Part model, mm, in its own coordinate system. Face numbers are marked on the shaded views. A direction names the side the tool comes from. Round coordinates to 2 decimals unless told otherwise and drop trailing zeros. Write each loop counter-clockwise with the first axis right and the second up, starting at its lowest first coordinate (ties: lowest second). Pieces come first, ordered by that corner, then holes.
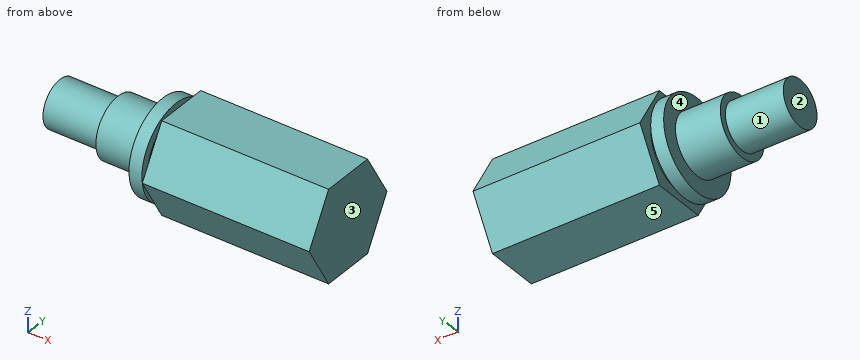
```python
from build123d import *

# Parameters (mm, degrees)
BOSS_EXTRUDE1_DEPTH = 22.86


with BuildPart() as part:
    # Sketch1 → Revolve1 (revolve)
    with BuildSketch(Plane.XY, mode=Mode.PRIVATE) as revolve1_sk:
        Polygon((0, 0), (0, 6.35), (-22.86, 6.35), (-22.86, 5.241687437), (-23.622, 5.241687437), (-23.622, 6.35), (-25.4, 6.35), (-25.4, 4.1275), (-31.5468, 4.1275), (-31.5468, 3.175), (-39.4843, 3.175), (-39.4843, 0), align=None)
    revolve(revolve1_sk.sketch.rotate(Axis((0, 0, 0), (-1, 0, 0)), 90), axis=Axis((0, 0, 0), (-1, 0, 0)))

    # Sketch2 → Boss-Extrude1 (add)
    with BuildSketch(Plane(origin=(0, 0, 0), x_dir=(0, 0, -1), z_dir=(1, 0, 0))):
        Polygon((-6.35, 3.666174209), (-6.35, -3.666174209), (0, -7.332348419), (6.35, -3.666174209), (6.35, 3.666174209), (0, 7.332348419), align=None)
    extrude(amount=-BOSS_EXTRUDE1_DEPTH)


solid = part.part
```
Q1. Wall check: L1, parallel to X at y = -5.5, z = 1; L2, parallel to X at y = 3.75, z = 0.25; L3, parallel to X at y = 1.75, z = 4.25. Give the ranges that are in metal, low to high.
Values follow:
L1: x = -25.4 to -23.62, -22.86 to 0
L2: x = -31.55 to 0
L3: x = -25.4 to 0
Q2. Which spindle directions (+Z, -Z, +X, -X, +Y, -Y) get a long thin tool onto all of the face, cutting with end or side? Do the marked faces 4 and 5. Say none if no direction does.
Values follow:
face 4: -X
face 5: -Z, +X, -X, +Y, -Y
Q3. Cut at C-C on z = -3.75. Write the cut outline in (x, y).
Values follow:
outline: (-31.55, -1.72) - (-25.4, -1.72) - (-25.4, -5.12) - (-23.62, -5.12) - (-23.62, -3.66) - (-22.86, -3.66) - (-22.86, -5.17) - (0, -5.17) - (0, 5.17) - (-22.86, 5.17) - (-22.86, 3.66) - (-23.62, 3.66) - (-23.62, 5.12) - (-25.4, 5.12) - (-25.4, 1.72) - (-31.55, 1.72) - close
Q4. Mould opens along X. For the marked faces 1, 2 and 3 say: +X half, -X half, draft (parallel to the pull), parting line (faces both ways), or undercut.
Values follow:
face 1: draft
face 2: -X half
face 3: +X half
Q5. Cut at D-D on y = -2.75. Write the cut outline in (x, z), plus the area to 3 significant figures.
Values follow:
outline: (-39.48, -1.59) - (-31.55, -1.59) - (-31.55, -3.08) - (-25.4, -3.08) - (-25.4, -5.72) - (-23.62, -5.72) - (-23.62, -4.46) - (-22.86, -4.46) - (-22.86, -6.35) - (0, -6.35) - (0, 6.35) - (-22.86, 6.35) - (-22.86, 4.46) - (-23.62, 4.46) - (-23.62, 5.72) - (-25.4, 5.72) - (-25.4, 3.08) - (-31.55, 3.08) - (-31.55, 1.59) - (-39.48, 1.59) - close
area: 381 mm2
Q6. Cut at A-A on x = -14. Write the cut outline in (y, z), plus the area to 3 significant figures.
Values follow:
outline: (-7.33, 0) - (-3.67, -6.35) - (3.67, -6.35) - (7.33, 0) - (3.67, 6.35) - (-3.67, 6.35) - close
area: 140 mm2
Q7. Drop flat-ended pins along their axis: pin 1 (2 mm diameter, centred on x = -26, z = 0, fed in from -Y); pin 2 (3 mm diameter, centred on y = -5, z = 1, fed in from -X); pin 3 (2 mm diameter, centred on x = -35, z = -2, fed in from +Y). Give the stop position or say it passes through.
Values follow:
pin 1: stops at y = -6.35
pin 2: stops at x = -31.55
pin 3: stops at y = 3.01
Q8. Cut at B-B on y = -0.75. Write the cut outline in (x, z), plus the area to 3 significant figures.
Values follow:
outline: (-39.48, -3.09) - (-31.55, -3.09) - (-31.55, -4.06) - (-25.4, -4.06) - (-25.4, -6.31) - (-23.62, -6.31) - (-23.62, -5.19) - (-22.86, -5.19) - (-22.86, -6.35) - (0, -6.35) - (0, 6.35) - (-22.86, 6.35) - (-22.86, 5.19) - (-23.62, 5.19) - (-23.62, 6.31) - (-25.4, 6.31) - (-25.4, 4.06) - (-31.55, 4.06) - (-31.55, 3.09) - (-39.48, 3.09) - close
area: 420 mm2
